Model file for the job. Use its own axes, mm. Face numbers are marked on the shaded views. A direction names the side the tool comes from. Round coordinates to 2 decimals unless told otherwise and drop trailing zeros. Write each loop counter-clockwise with the first axis right and the second up, starting at its lowest first coordinate (ties: lowest second). Pieces come first, ordered by that corner, then holes. Notation, with made-up numbers: (70, -10) - (123, -10) arc R25 ccw to (123, 19) - close; hole circle Ø10 at (-29, 79). An arc over 180 degrees is marked (long way). Answer as a JSON object with one key per item and string values. Group by question number.
from build123d import *

# Parameters (mm, degrees)
PAD_DEPTH       = 15
SKETCH001_W     = 23
SKETCH001_H     = 33
POCKET_DEPTH    = 13
SKETCH002_R     = 1.5
HOLE_DEPTH      = 25
POCKET001_DEPTH = 8
POCKET002_DEPTH = 5
SKETCH006_W     = 7
SKETCH006_H     = 8
POCKET004_DEPTH = 5
SKETCH007_W     = 3
SKETCH007_H     = 2
POCKET005_DEPTH = 50
POCKET006_DEPTH = 50
FILLET_R        = 0.7
POCKET008_DEPTH = 14
SKETCH009_W     = 4
SKETCH009_H     = 9
POCKET009_DEPTH = 6.5
FILLET001_R     = 0.7
FILLET002_R     = 0.7


with BuildPart() as part:
    # Sketch → Pad (new body)
    with BuildSketch(Plane.XY):
        with BuildLine():
            ThreePointArc((14.5, 46), (15.56066, 46.43934), (16, 47.5))
            Line((16, 47.5), (16, 65))
            ThreePointArc((16, 65), (14.242641, 69.242641), (10, 71))
            Line((-10, 71), (10, 71))
            ThreePointArc((-10, 71), (-14.242641, 69.242641), (-16, 65))
            Line((-16, 47.5), (-16, 65))
            ThreePointArc((-16, 47.5), (-15.56066, 46.43934), (-14.5, 46))
            Line((-13.5, 46), (-14.5, 46))
            ThreePointArc((-13.5, 40), (-10.5, 43), (-13.5, 46))
            Line((-13.5, 40), (-14.5, 40))
            ThreePointArc((-14.5, 40), (-15.56066, 39.56066), (-16, 38.5))
            Line((-16, 3), (-16, 38.5))
            ThreePointArc((-16, 3), (-15.12132, 0.87868), (-13, 0))
            Line((13, 0), (-13, 0))
            ThreePointArc((13, 0), (15.12132, 0.87868), (16, 3))
            Line((16, 3), (16, 38.5))
            ThreePointArc((16, 38.5), (15.56066, 39.56066), (14.5, 40))
            Line((14.5, 40), (13.5, 40))
            ThreePointArc((13.5, 46), (10.5, 43), (13.5, 40))
            Line((14.5, 46), (13.5, 46))
        make_face()
    extrude(amount=PAD_DEPTH)

    # Sketch001 (on Face22 of Pad) → Pocket (cut)
    with BuildSketch(Plane.XY.offset(15)):
        with Locations((0, 19.5)):
            Rectangle(SKETCH001_W, SKETCH001_H)
        with BuildLine():
            Line((-4.010044, 65.347033), (-2.994978, 47.826484))
            ThreePointArc((-2.994978, 47.826484), (0, 45), (2.994978, 47.826484))
            Line((4.010044, 65.347033), (2.994978, 47.826484))
            ThreePointArc((10, 71), (5.881881, 69.363611), (4.010044, 65.347033))
            Line((10, 74.59), (10, 71))
            Line((-10, 74.59), (10, 74.59))
            Line((-10, 71), (-10, 74.59))
            ThreePointArc((-4.010044, 65.347033), (-5.881881, 69.363611), (-10, 71))
        make_face()
    extrude(amount=-POCKET_DEPTH, mode=Mode.SUBTRACT)

    # Sketch002 (on Face5 of Pocket) → Hole (cut)
    with BuildSketch(Plane.XY.offset(15)):
        with Locations((-10, 65)):
            Circle(SKETCH002_R)
        with Locations((10, 65)):
            Circle(SKETCH002_R)
        with Locations((-10, 51.5)):
            Circle(SKETCH002_R)
        with Locations((10, 51.5)):
            Circle(SKETCH002_R)
    extrude(amount=-HOLE_DEPTH, mode=Mode.SUBTRACT)

    # Sketch003 (on Face5 of Hole) → Pocket001 (cut)
    with BuildSketch(Plane.XY.offset(15)):
        Polygon((-7, 63.267949), (-7, 66.732051), (-10, 68.464102), (-13, 66.732051), (-13, 63.267949), (-10, 61.535898), align=None)
        Polygon((-7, 49.767949), (-7, 53.232051), (-10, 54.964102), (-13, 53.232051), (-13, 49.767949), (-10, 48.035898), align=None)
        Polygon((13, 49.767949), (13, 53.232051), (10, 54.964102), (7, 53.232051), (7, 49.767949), (10, 48.035898), align=None)
        Polygon((13, 63.267949), (13, 66.732051), (10, 68.464102), (7, 66.732051), (7, 63.267949), (10, 61.535898), align=None)
    extrude(amount=-POCKET001_DEPTH, mode=Mode.SUBTRACT)

    # Sketch004 (on Face65 of Pocket001) → Pocket002 (cut)
    with BuildSketch(Plane.XY.offset(2)):
        Polygon((-11.5, 5), (-3.5, 5), (-3.5, 6), (11.5, 6), (11.5, 28), (9, 28), (9, 34), (-9, 34), (-9, 14), (-11.5, 14), align=None)
    extrude(amount=-POCKET002_DEPTH, mode=Mode.SUBTRACT)

    # Sketch006 → Pocket004 (cut)
    with BuildSketch(Plane.XZ):
        with Locations((4.5, 6)):
            Rectangle(SKETCH006_W, SKETCH006_H)
    extrude(amount=-POCKET004_DEPTH, mode=Mode.SUBTRACT)

    # Sketch007 (on Face12 of Pocket004) → Pocket005 (cut)
    with BuildSketch(Plane.YZ.offset(16)):
        with Locations((4.5, 6.5)):
            Rectangle(SKETCH007_W, SKETCH007_H)
        with Locations((34.5, 7.5)):
            Rectangle(SKETCH007_W, SKETCH007_H)
    extrude(amount=-POCKET005_DEPTH, mode=Mode.SUBTRACT)

    # Sketch008 (on Face12 of Pocket005) → Pocket006 (cut)
    with BuildSketch(Plane.YZ.offset(16)):
        Polygon((0, 10), (10, 10), (38.5, 15), (47.5, 15), (65, 10), (71, 10), (71, 16.83), (0, 16.83), align=None)
    extrude(amount=-POCKET006_DEPTH, mode=Mode.SUBTRACT)

    # Fillet
    fillet_edges = [part.edges().sort_by_distance(p)[0] for p in [
        (-9, 14, 1),
        (-11.5, 14, 1),
    ]]
    fillet(fillet_edges, radius=FILLET_R)

    # MirroredSketch → Pocket008 (cut)
    with BuildSketch(Plane.XY.offset(15)):
        with BuildLine():
            Line((2.5, 30), (-10.5, 30))
            ThreePointArc((-11.5, 31), (-11.207107, 30.292893), (-10.5, 30))
            Line((-11.5, 31), (-11.5, 35.5))
            ThreePointArc((-11, 36), (-11.353553, 35.853553), (-11.5, 35.5))
            Line((-11, 36), (-10.99, 36))
            ThreePointArc((-10.99, 36), (-10.636447, 36.146447), (-10.49, 36.5))
            Line((-10.49, 36.5), (-10.49, 38.675662))
            ThreePointArc((-10.49, 38.675662), (-9.67833, 39.262821), (-9, 40))
            Line((1.49, 40), (-9, 40))
            ThreePointArc((2.49, 39), (2.197107, 39.707107), (1.49, 40))
            Line((2.49, 36.5), (2.49, 39))
            ThreePointArc((2.49, 36.5), (2.636447, 36.146447), (2.99, 36))
            Line((3, 36), (2.99, 36))
            ThreePointArc((3.5, 35.5), (3.353553, 35.853553), (3, 36))
            Line((3.5, 31), (3.5, 35.5))
            ThreePointArc((2.5, 30), (3.207107, 30.292893), (3.5, 31))
        make_face()
    extrude(amount=-POCKET008_DEPTH, mode=Mode.SUBTRACT)

    # Sketch009 (on Face88 of Pocket008) → Pocket009 (cut, symmetric)
    with BuildSketch(Plane.XZ.offset(-40)):
        with Locations((0, 6.5)):
            Rectangle(SKETCH009_W, SKETCH009_H)
    extrude(amount=POCKET009_DEPTH, both=True, mode=Mode.SUBTRACT)

    # Fillet001
    fillet001_edges = [part.edges().sort_by_distance(p)[0] for p in [
        (9, 28, 1),
    ]]
    fillet(fillet001_edges, radius=FILLET001_R)

    # Fillet002
    fillet002_edges = [part.edges().sort_by_distance(p)[0] for p in [
        (-3.5, 6, 1),
    ]]
    fillet(fillet002_edges, radius=FILLET002_R)


solid = part.part
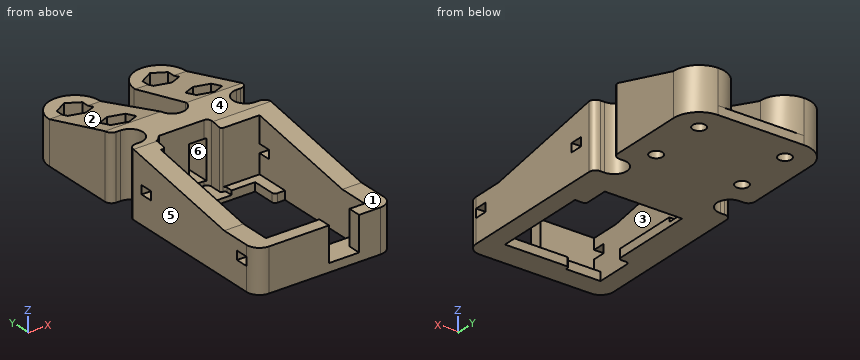
(1) 3-axis set-ups, long thin cutter, end or side, ignore diameter. For the marked faces 1, 2 and 3: which of +Z, -Z, +X, -X, +Y, -Y reach the whole face in a straight line?
(2) Pull direction X, two halves, no side cores. Call the marked faces 4, 5 and 6: pulls with the +X half, pulls with the -X half, needs draft (parallel to the pull), parting line crosses it, or undercut.
(3) Slice it at B-B (z = 4.5). Count the separate pieces of the cut face and the enclosed holes in it, then the cut area to 3 significant figures.
(4) Slice it at A-A (x = 0). Write the cut outline in (y, z), then the cut area to 3 significant figures.
(5) Slice it at D-D (y = 57.5). Write the cut outline in (x, z).
(6) Flat gauge pins, fed straight in: pin 1 (1 mm diameter, centred on x = -15, z = 7.5, fed in from +Y); pin 2 (1.8 mm diameter, centred on x = -7.5, y = 68.5, fed in from +Z); pin 3 (0.9 mm diameter, centred on x = -13.5, y = 5, fed in from -Z); pin 4 (10 mm diameter, centred on x = 4.5, y = 58, fed in from +Z). Where does each tip first touch, or does it go through?
(7) Slice it at C-C (x = 5.5). Write the cut outline in (y, z), then the cut area to 3 significant figures.
(8) Drill centre lines: line 1 (X direction, y = 65, z = 2.5); line 2 (Y direction, x = 10, z = 3); line 3 (Y direction, x = 10, z = 10.25). Where is each one in solid material? Low to high. Write a range as from..to.
Answer:
{
 "1": {"face 1": "+Z, +X, -X, -Y", "face 2": "+Z, +X, -X, +Y", "face 3": "+Z"},
 "2": {"face 4": "needs draft", "face 5": "pulls with the -X half", "face 6": "undercut"},
 "3": {"separate pieces": "2", "enclosed holes": "4", "area": "1,120 mm²"},
 "4": {"outline": "(0, 0) - (6, 0) - (6, 2) - (3, 2) - (3, 10) - (0, 10) - close; (34, 0) - (71, 0) - (71, 2) - (40, 2) - (40, 1) - (34, 1) - close; (40, 11) - (45, 11) - (45, 15) - (40, 15) - close", "area": "124 mm²"},
 "5": {"outline": "(-16, 0) - (16, 0) - (16, 12.14) - (3.56, 12.14) - (3.56, 2) - (-3.56, 2) - (-3.56, 12.14) - (-16, 12.14) - close"},
 "6": {"pin 1": "y = 68.97", "pin 2": "z = 10", "pin 3": "z = 0", "pin 4": "z = 13.43"},
 "7": {"outline": "(0, 0) - (6, 0) - (6, 2) - (0, 2) - close; (34, 0) - (71, 0) - (71, 2) - (68.97, 2) - (68.97, 10) - (65, 10) - (47.5, 15) - (38.5, 15) - (36, 14.56) - (36, 2) - (34, 2) - close", "area": "450 mm²"},
 "8": {"line 1": "-16..-11.5, -8.5..-3.99, 3.99..8.5, 11.5..16", "line 2": "0..3, 36..50, 53..63.5, 66.5..71", "line 3": "36..48.04, 54.96..61.54"}
}
